from build123d import *

# Parameters (mm, degrees)
F1_DEPTH = 10
F2_D     = 8
F3_D     = 8
F4_D     = 8
F5_D     = 8
F6_W     = 30
F6_H     = 66.012212
F7_DEPTH = 40


with BuildPart() as f1:
    # F0 (on Top) → F1 (new body)
    with BuildSketch(Plane.XY):
        with BuildLine():
            Line((30, 35), (-30, 35))
            ThreePointArc((-30, 35), (-31.767767, 34.267767), (-32.5, 32.5))
            Line((-32.5, 32.5), (-32.5, -32.5))
            ThreePointArc((-32.5, -32.5), (-31.767767, -34.267767), (-30, -35))
            Line((-30, -35), (30, -35))
            ThreePointArc((30, -35), (31.767767, -34.267767), (32.5, -32.5))
            Line((32.5, -32.5), (32.5, 32.5))
            ThreePointArc((32.5, 32.5), (31.767767, 34.267767), (30, 35))
        make_face()
    extrude(amount=F1_DEPTH)

    # F2 (through all)
    with Locations(Plane(origin=(0, 0, 0), x_dir=(1, 0, 0), z_dir=(0, 0, -1))):
        with Locations((24.5, 27)):
            Hole(F2_D / 2)

    # F3 (through all)
    with Locations(Plane(origin=(0, 0, 0), x_dir=(1, 0, 0), z_dir=(0, 0, -1))):
        with Locations((-24.5, 27)):
            Hole(F3_D / 2)

    # F4 (through all)
    with Locations(Plane(origin=(0, 0, 0), x_dir=(1, 0, 0), z_dir=(0, 0, -1))):
        with Locations((24.5, -27)):
            Hole(F4_D / 2)

    # F5 (through all)
    with Locations(Plane(origin=(0, 0, 0), x_dir=(1, 0, 0), z_dir=(0, 0, -1))):
        with Locations((-24.5, -27)):
            Hole(F5_D / 2)

    # F6 (on Top) + F0 (on Top) → F7 (join)
    with BuildSketch(Plane.XY):
        Rectangle(F6_W, F6_H)
    with BuildSketch(Plane.XY):
        with BuildLine():
            Line((30, 35), (-30, 35))
            ThreePointArc((-30, 35), (-31.767767, 34.267767), (-32.5, 32.5))
            Line((-32.5, 32.5), (-32.5, -32.5))
            ThreePointArc((-32.5, -32.5), (-31.767767, -34.267767), (-30, -35))
            Line((-30, -35), (30, -35))
            ThreePointArc((30, -35), (31.767767, -34.267767), (32.5, -32.5))
            Line((32.5, -32.5), (32.5, 32.5))
            ThreePointArc((32.5, 32.5), (31.767767, 34.267767), (30, 35))
        make_face()
    extrude(amount=-F7_DEPTH)


solid = f1.part
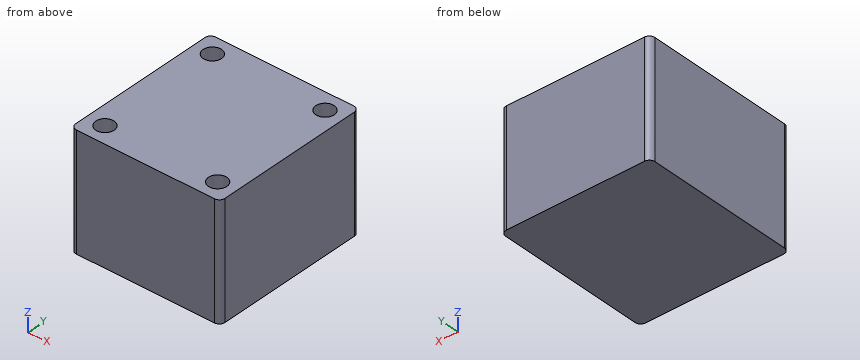
Build history of the part. All positions in model axes, mm. Give positions to 0.01 mm unless a question says otherwise; leave off trailing zeros. Order: outer loops, then holes, each group sorted by start corner. A loop starts at its lowest first (then second) coordinate and runs counter-clockwise, first axis right, second up. Notation, with made-up numbers: M 39,24 L 64,24 A9 cw 64,32 Z; hole C -17,88 d6. An arc over 180 degrees is marked long. Use one line per item in the form item = value.
Q1. Wall check: probe 1 along Y at (x, z) = (24.5, 4.5); probe 2 along X at (y, z) = (-27, 3). Give the ranges that are in metal, low to high.
Conclusion:
probe_1 = -35 to -31, -23 to 23, 31 to 35
probe_2 = -32.5 to -28.5, -20.5 to 20.5, 28.5 to 32.5
Q2. Slice it at A-A, the plane x = 24.5. Write the cut outline in (y, z).
Conclusion:
outline = M -35,-40 L 35,-40 L 35,10 L 31,10 L 31,0 L 23,0 L 23,10 L -23,10 L -23,0 L -31,0 L -31,10 L -35,10 Z
Q3. Slice it at B-B, the plane y = 27. Write the cut outline in (x, z).
Conclusion:
outline = M -32.5,-40 L 32.5,-40 L 32.5,10 L 28.5,10 L 28.5,0 L 20.5,0 L 20.5,10 L -20.5,10 L -20.5,0 L -28.5,0 L -28.5,10 L -32.5,10 Z
Q4. Pin check, flat tip, straight feed: P1, Ø2.5, axis at x = -26, y = 25.5, coming from the +Z side. Stop position of the tip, or through.
Conclusion:
P1 = 0
